```python
from build123d import *

# Parameters (mm, degrees)
BOSS_EXTRUDE1_DEPTH      = 304.8
BOSS_EXTRUDE1_DEPTH_BACK = 304.8
CUT_EXTRUDE1_DEPTH       = 26.4


with BuildPart() as part:
    # Sketch1 → Boss-Extrude1 (new body, two sides)
    with BuildSketch(Plane.XY) as boss_extrude1_sk:
        Polygon((0, 25.4), (0, 0), (25.4, 0), (25.4, 1.27), (1.27, 1.27), (1.27, 25.4), align=None)
    extrude(amount=BOSS_EXTRUDE1_DEPTH)
    extrude(boss_extrude1_sk.sketch, amount=-BOSS_EXTRUDE1_DEPTH_BACK)

    # Sketch2 → Cut-Extrude1 (cut, through all)
    with BuildSketch(Plane.ZY):
        Polygon((223.77, 0), (198.37, 25.4), (304.8, 25.4), (304.8, 0), align=None)
        Polygon((-304.8, 0), (-304.8, 25.4), (-198.37, 25.4), (-223.77, 0), align=None)
    extrude(amount=-CUT_EXTRUDE1_DEPTH, mode=Mode.SUBTRACT)


solid = part.part
```
Design review of the part built by this model. Coordinates are the model's own, in mm. A direction names the side the tool comes from. Give positions to 0.01 mm unless a question says otherwise; leave off trailing zeros. Write each loop counter-clockwise with the first axis right and the second up, starting at its lowest first coordinate (ties: lowest second). Pieces come first, ordered by that corner, then holes. Notation, with made-up numbers: (12.25, -13) -> (54.25, -13) arc R20 ccw to (54.25, -2) -> close; hole circle Ø8 at (46.5, 85). An arc over 180 degrees is marked (long way). Answer in a Markdown table with one row per item.
(1) For faces 1 (the flat face through (14, 1.27, 3)), 2 (the flat face through (0, 13, 3)), list the 3-axis set-ups (+Z, -Z, +X, -X, +Y, -Y) from which the entire face can be reached by the end or side of a thin tool; tool diameter is ignored.
Results:
| item | result |
|---|---|
| face 1 | +Z, -Z, +X, +Y |
| face 2 | +Z, -Z, -X, +Y, -Y |
(2) Consider section B-B (z = 87). State the section outline as (x, y) points.
Results:
| item | result |
|---|---|
| outline | (0, 0) -> (25.4, 0) -> (25.4, 1.27) -> (1.27, 1.27) -> (1.27, 25.4) -> (0, 25.4) -> close |
(3) To check wall thickness, follow probe 1 along X at (y, z) = (12, 121). State the ranges of the line that lie inside material, in increasing order.
Results:
| item | result |
|---|---|
| probe 1 | 0 to 1.27 |
(4) Consider section A-A (y = 12.5). State the section outline as (x, z) points, then the cut area to 3 significant figures.
Results:
| item | result |
|---|---|
| outline | (0, -211.27) -> (1.27, -211.27) -> (1.27, 211.27) -> (0, 211.27) -> close |
| area | 537 mm2 |
(5) Consider section C-C (x = 5.5). State the section outline as (y, z) points, then the cut area to 3 significant figures.
Results:
| item | result |
|---|---|
| outline | (0, -223.77) -> (1.27, -222.5) -> (1.27, 222.5) -> (0, 223.77) -> close |
| area | 567 mm2 |
(6) Clearance check with flat-ended pins moving along their axes: pin 1 (12 mm diameter, centred on x = 16, z = 45, fed in from +Y); pin 2 (6 mm diameter, centred on y = 5.5, z = 100, fed in from +X). State where each tip first meets the part, or that it passes through.
Results:
| item | result |
|---|---|
| pin 1 | y = 1.27 |
| pin 2 | x = 1.27 |
